```python
from build123d import *

# Parameters (mm, degrees)
BOSS_EXTRUDE1_DEPTH = 10
SKETCH2_R           = 2.25
CUT_EXTRUDE1_DEPTH  = 28.49545417
SKETCH3_W           = 39
SKETCH3_H           = 5
BOSS_EXTRUDE2_DEPTH = 10
SKETCH4_R           = 1.75
CUT_EXTRUDE2_DEPTH  = 27.55654345
CUT_EXTRUDE3_DEPTH  = 1
BOSS_EXTRUDE3_START = 0.75
SKETCH5_R           = 4
SKETCH5_R_2         = 2.25
BOSS_EXTRUDE3_DEPTH = 0.75
FILLET1_R           = 1
SKETCH7_R           = 1.75
CUT_EXTRUDE4_DEPTH  = 2


with BuildPart() as part:
    # Sketch1 → Boss-Extrude1 (new body)
    with BuildSketch(Plane(origin=(0, 0, 0), x_dir=(1, 0, 0), z_dir=(0, 1, 0))):
        Polygon((8, 0), (0, 0), (0, -5), (5, -5), (5, -20), (8, -20), align=None)
        Polygon((0, -5), (0, 0), (-8, 0), (-8, -20), (-5, -20), (-5, -5), align=None)
    extrude(amount=BOSS_EXTRUDE1_DEPTH)

    # Sketch2 → Cut-Extrude1 (cut, through all)
    with BuildSketch(Plane(origin=(8, 0, 0), x_dir=(0, 0, -1), z_dir=(1, 0, 0))):
        with Locations((-13, 5)):
            Circle(SKETCH2_R)
    extrude(amount=-CUT_EXTRUDE1_DEPTH, mode=Mode.SUBTRACT)

    # Sketch3 → Boss-Extrude2 (add, through all)
    with BuildSketch(Plane(origin=(0, 10, 0), x_dir=(1, 0, 0), z_dir=(0, 1, 0))):
        with Locations((0, -2.5)):
            Rectangle(SKETCH3_W, SKETCH3_H)
    extrude(amount=-BOSS_EXTRUDE2_DEPTH)

    # Sketch4 → Cut-Extrude2 (cut, through all)
    with BuildSketch(Plane.XY.offset(5)):
        with Locations((-15, 5)):
            Circle(SKETCH4_R)
        with Locations(Location((15, 5, 0), (0, 0, 180))):
            Circle(SKETCH4_R)
    extrude(amount=-CUT_EXTRUDE2_DEPTH, mode=Mode.SUBTRACT)

    # Sketch6 → Cut-Extrude3 (cut)
    with BuildSketch(Plane(origin=(-5, 0, 0), x_dir=(0, 0, -1), z_dir=(1, 0, 0))):
        with BuildLine():
            Line((-13, 12.5), (-20.5, 12.5))
            Line((-20.5, 12.5), (-20.5, 5))
            Line((-20.5, 5), (-20.5, -2.5))
            Line((-20.5, -2.5), (-13, -2.5))
            ThreePointArc((-13, -2.5), (-5.5, 5), (-13, 12.5))
        make_face()
    cut_extrude3 = extrude(amount=-CUT_EXTRUDE3_DEPTH, mode=Mode.SUBTRACT)

    # Sketch5 → Boss-Extrude3 (add)
    with BuildSketch(Plane(origin=(-6, 0, 0), x_dir=(0, 0, -1), z_dir=(1, 0, 0)).offset(BOSS_EXTRUDE3_START)):
        with Locations((-13, 5)):
            Circle(SKETCH5_R)
        with Locations((-13, 5)):
            Circle(SKETCH5_R_2, mode=Mode.SUBTRACT)
    boss_extrude3 = extrude(amount=-BOSS_EXTRUDE3_DEPTH)

    # Mirror1: Cut-Extrude3, Boss-Extrude3 across plane
    add(cut_extrude3.mirror(Plane(origin=(0, 0, 0), x_dir=(0, 0, 1), z_dir=(1, 0, 0))), mode=Mode.SUBTRACT)
    add(boss_extrude3.mirror(Plane(origin=(0, 0, 0), x_dir=(0, 0, 1), z_dir=(1, 0, 0))))

    # Fillet1
    fillet1_edges = [part.edges().sort_by_distance(p)[0] for p in [
        (-6, 5, 5.5),
        (6, 5, 5.5),
        (5, 5, 5),
        (-5, 5, 5),
        (8, 5, 5),
        (-8, 5, 5),
    ]]
    fillet(fillet1_edges, radius=FILLET1_R - 0.0001)  # a hair under: the kernel refuses the full size

    # Sketch7 → Cut-Extrude4 (cut)
    # profile 1 of 3: a face of its own
    with BuildSketch(Plane.XY.offset(5)):
        Polygon((-16.804219591, 8.125), (-13.195780409, 8.125), (-11.391560818, 5), (-13.195780409, 1.875), (-16.804219591, 1.875), (-18.608439182, 5), align=None)
    # profile 2 of 3: a face of its own
    with BuildSketch(Plane.XY.offset(5)):
        Polygon((16.804219591, 1.875), (18.608439182, 5), (16.804219591, 8.125), (13.195780409, 8.125), (11.391560818, 5), (13.195780409, 1.875), align=None)
        with Locations((15, 5)):
            Circle(SKETCH7_R, mode=Mode.SUBTRACT)
    # profile 3 of 3: a face of its own
    with BuildSketch(Plane.XY.offset(5)):
        with Locations((15, 5)):
            Circle(SKETCH7_R)
    extrude(amount=-CUT_EXTRUDE4_DEPTH, mode=Mode.SUBTRACT)


solid = part.part
```
The listing builds one solid part. Answer for the finished solid, in the listing's coordinates (mm). A direction names the side the tool comes from. Coordinates: 2 decimals unless noted, no trailing zeros. Write each loop counter-clockwise with the first axis right and the second up, starting at its lowest first coordinate (ties: lowest second). Pieces come first, ordered by that corner, then holes. Notation, with made-up numbers: M 73,-14 L 122,-14 A18 ccw 122,2 Z; hole C 7.25,-31.5 d7. An arc over 180 degrees is marked long. Use a Markdown table: item, result. Add a question column.
1. Which of the six approach directions +Z, -Z, +X, -X, +Y, -Y give full straight-line access (tool end or side, diameter ignored) to faces 1 (the flat face through (6, 5, 18)), 2 (the flat face through (15, 1.875, 4)), 3 (the cylindrical face through (6.61, 6.52, 14.66)), 4 (the flat face through (-8, 3, 11)), 5 (the flat face through (-5, 0.6, 6.4))?
2. Section B-B (x = -15) is taken. Give the vertices of the cut face in (y, z) (3 decimals), plus the area to 3 significant figures.
3. Section A-A (z = 13) is taken. Give the vertices of the cut face in (x, y).
4. Given P1, Ø3, axis at x = -15.5, y = 4, coming from the +Z side; P2, Ø3, axis at y = 6, z = 12, coming from the -X side; P3, Ø5, axis at x = 12.5, y = 9, coming from the +Z side, each flat-ended and moving along its own axis, determine where each tip first touches the part or whether it passes through.
5. For a pull along X with two mould halves and no side action, classify faces 6 (the flat face through (-13, 6, 3)), 7 (the flat face through (0, 5, 0)), 8 (the cylindrical face through (-8.301, 4.93, 5.285)) as +X half, -X half, draft (parallel to the pull), parting line (faces both ways), or undercut.
6. Section C-C (z = 18.25) is taken. Give the vertices of the cut face in (x, y), plus the area to 3 significant figures.
7. Section D-D (x = -11) is taken. Give the vertices of the cut face in (y, z), plus the area to 3 significant figures.
8. Straight lines are drawn through the part: line 1 along X through (y, z) = (7, 11.75); line 2 along Y through (x, z) = (6.1, 13); line 3 along X through (y, z) = (6, 17). For each, find the intervals that lie inside material, in ascending order. Write a range as [from, to].
Data:
| question | item | result |
|---|---|---|
| 1 | face 1 | none |
| 1 | face 2 | +Z |
| 1 | face 3 | +X, -X |
| 1 | face 4 | +Z, -X, +Y, -Y |
| 1 | face 5 | +Z, +Y, -Y |
| 2 | outline | M 0,0 L 3.25,0 L 3.25,3 L 1.875,3 L 1.875,5 L 0,5 Z; M 6.75,0 L 10,0 L 10,5 L 8.125,5 L 8.125,3 L 6.75,3 Z |
| 2 | area | 27.0 mm2 |
| 3 | outline | M -8,0 L -6,0 L -6,1 L -5.25,1 L -5.25,2.75 L -8,2.75 Z; M -8,7.25 L -5.25,7.25 L -5.25,9 L -6,9 L -6,10 L -8,10 Z; M 5.25,1 L 6,1 L 6,0 L 8,0 L 8,2.75 L 5.25,2.75 Z; M 5.25,7.25 L 8,7.25 L 8,10 L 6,10 L 6,9 L 5.25,9 Z |
| 4 | P1 | stops at z = 3 |
| 4 | P2 | stops at x = -8 |
| 4 | P3 | stops at z = 5 |
| 5 | face 6 | undercut |
| 5 | face 7 | draft |
| 5 | face 8 | -X half |
| 6 | outline | M -8,0 L -6,0 L -6,10 L -8,10 Z; M 6,0 L 8,0 L 8,10 L 6,10 Z |
| 6 | area | 40.0 mm2 |
| 7 | outline | M 0,0 L 10,0 L 10,5 L 0,5 Z |
| 7 | area | 50.0 mm2 |
| 8 | line 1 | x = [-8, -5.25], [5.25, 8] |
| 8 | line 2 | y = [0, 2.75], [7.25, 10] |
| 8 | line 3 | x = [-8, -6], [6, 8] |
